Could you check a few things on this model? Use its own coordinates, in mm. Face numbers are marked on the shaded views. A direction names the side the tool comes from. Give positions to 0.01 mm unless a question says otherwise; leave off trailing zeros. Order: outer loops, then holes, each group sorted by start corner. A loop starts at its lowest first (then second) coordinate and runs counter-clockwise, first axis right, second up. Notation, with made-up numbers: (37.5, 22.5) -> (59.5, 22.5) arc R26 cw to (59.5, 56.5) -> close; hole circle Ø1 at (32, 49). An arc over 180 degrees is marked (long way). Answer as CSV lines item,"result". Start each with the question number.
(1) I want a section at B-B (z = 13). Please give me the cut outline in (x, y).
(2) On a 3-axis mill with a long thin cutter (end or side, diameter ignored), from which of +Z, -Z, +X, -X, +Y, -Y can I reach the whole of each face in a straight line? I mean the marked faces 1 and 2. Say none if no direction works.
(3) Will these pins go through, and if not, where does the flat tip stop? pin 1 Ø5 at (x, z) = (-13.5, 4) entering from +Y; pin 2 Ø3 at (y, z) = (-15, 28) entering from +X; pin 3 Ø2 at (y, z) = (9.5, 14) entering from -X; pin 4 Ø6 at (y, z) = (0, 14) entering from +X.
(4) We'd pull the mould along Y, two halves only. Please class the marked faces 3, 4 and 5: released by +Y, released by -Y, zero draft, split by the parting line, or undercut.
(5) I want a section at D-D (x = -21.5). Please give me the cut outline in (y, z), plus the area to 3 significant figures.
(6) I want a section at A-A (y = 0). Please give me the cut outline in (x, z), plus the area to 3 significant figures.
(7) I need wall thicknesses on L1, parallel to Y at x = 0, z = 16.5; L2, parallel to Y at x = 10.5, z = 31.5; L3, parallel to X at y = 15.5, z = 14.5. Which ranges of each line are inside material? Lowest first, please.
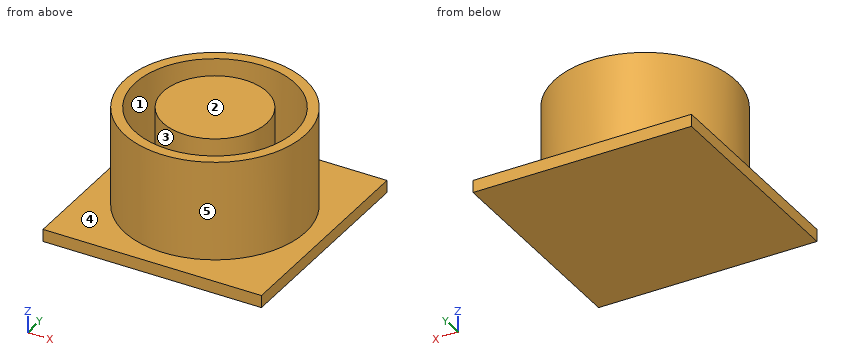
```python
from build123d import *

# Parameters (mm, degrees)
SKETCH1_W           = 70.29196
SKETCH1_H           = 70.29196
BOSS_EXTRUDE1_DEPTH = 3.9624
BOSS_EXTRUDE2_START = 3.9624
SKETCH1_3_R         = 29.111326452
SKETCH1_3_R_2       = 25.7683
BOSS_EXTRUDE2_DEPTH = 32.0294
BOSS_EXTRUDE3_START = 3.9624
SKETCH1_4_R         = 16.7259
BOSS_EXTRUDE3_DEPTH = 32.0294


with BuildPart() as part:
    # Sketch1 → Boss-Extrude1 (new body)
    with BuildSketch(Plane.XY):
        Rectangle(SKETCH1_W, SKETCH1_H)
    extrude(amount=BOSS_EXTRUDE1_DEPTH)

    # Sketch1<3> → Boss-Extrude2 (add)
    with BuildSketch(Plane.XY.offset(BOSS_EXTRUDE2_START)):
        Circle(SKETCH1_3_R)
        Circle(SKETCH1_3_R_2, mode=Mode.SUBTRACT)
    extrude(amount=BOSS_EXTRUDE2_DEPTH)

    # Sketch1<4> → Boss-Extrude3 (add)
    with BuildSketch(Plane.XY.offset(BOSS_EXTRUDE3_START)):
        Circle(SKETCH1_4_R)
    extrude(amount=BOSS_EXTRUDE3_DEPTH)


solid = part.part
```
Final values:
1,outline,"circle Ø58.22 at (0, 0); circle Ø33.45 at (0, 0); hole circle Ø51.54 at (0, 0)"
2,face 1,"+Z"
2,face 2,"+Z, +X, -X, +Y, -Y"
3,pin 1,"y = 35.15"
3,pin 2,"x = 25.79"
3,pin 3,"x = -27.84"
3,pin 4,"x = 29.11"
4,face 3,"undercut"
4,face 4,"zero draft"
4,face 5,"split by the parting line"
5,outline,"(-35.15, 0) -> (35.15, 0) -> (35.15, 3.96) -> (19.63, 3.96) -> (19.63, 35.99) -> (14.2, 35.99) -> (14.2, 3.96) -> (-14.2, 3.96) -> (-14.2, 35.99) -> (-19.63, 35.99) -> (-19.63, 3.96) -> (-35.15, 3.96) -> close"
5,area,"626 mm²"
6,outline,"(-35.15, 0) -> (35.15, 0) -> (35.15, 3.96) -> (29.11, 3.96) -> (29.11, 35.99) -> (25.77, 35.99) -> (25.77, 3.96) -> (16.73, 3.96) -> (16.73, 35.99) -> (-16.73, 35.99) -> (-16.73, 3.96) -> (-25.77, 3.96) -> (-25.77, 35.99) -> (-29.11, 35.99) -> (-29.11, 3.96) -> (-35.15, 3.96) -> close"
6,area,"1,560 mm²"
7,L1,"-29.11 to -25.77, -16.73 to 16.73, 25.77 to 29.11"
7,L2,"-27.15 to -23.53, -13.02 to 13.02, 23.53 to 27.15"
7,L3,"-24.64 to -20.59, -6.29 to 6.29, 20.59 to 24.64"
